Geometry check sheet. Reference: drawing and pictorial views, mm from the part's lowest x, y, z. A direction names the side the tool comes from. Coordinates: 2 decimals unless noted, no trailing zeros. Write each loop counter-clockwise with the first axis right and the second up, starting at its lowest first coordinate (ties: lowest second). Pieces come first, ordered by that corner, then holes. Notation, with made-up numbers: M -38,89 L 5,89 A31 cw 5,122 Z; hole C 49,-28.5 d11. An arc over 180 degrees is marked long. One line per item, written item: value.
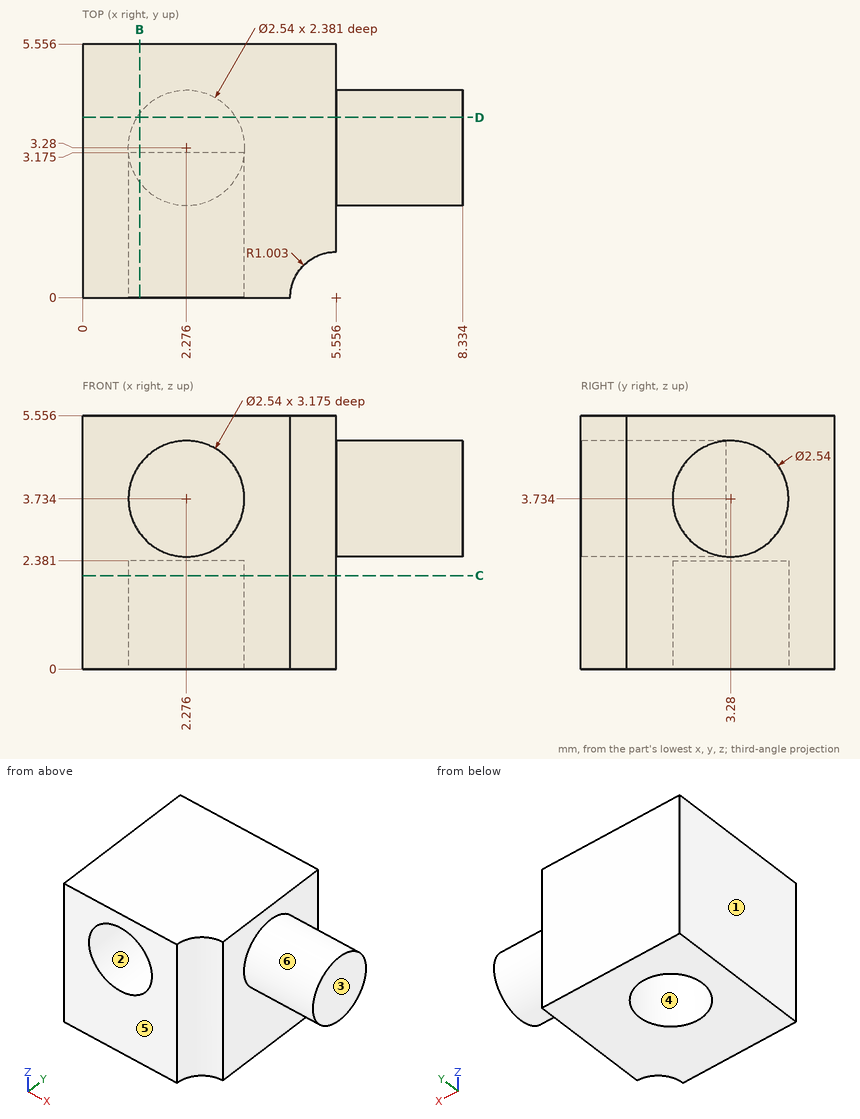
Item 1: Cross-section at D-D, the plane y = 3.95. Enter the section's corners in (x, z) (1 decimal).
The answers:
outline: M 0,0 L 1.2,0 L 1.2,2.4 L 3.4,2.4 L 3.4,0 L 5.6,0 L 5.6,2.7 L 8.3,2.7 L 8.3,4.8 L 5.6,4.8 L 5.6,5.6 L 0,5.6 Z
Item 2: Go/stop test with flat-tipped pins: P1, Ø1, axis at y = 5, z = 3.5, coming from the +X side; P2, Ø3, axis at y = 2.5, z = 1, coming from the +X side. Record where each tip stops, or that it passes through.
The answers:
P1: stops at x = 8.33
P2: stops at x = 5.56
Item 3: Scan lines: line 1 (Y direction, x = 3, z = 4.7) (1 decimal); line 2 (Y direction, x = 3.25, z = 2.2) (1 decimal); line 3 (X direction, y = 1.9, z = 4.35) (1 decimal). Record each from-to range of solid material in increasing order.
The answers:
line 1: y = 3.2 to 5.6
line 2: y = 0 to 2.5, 4.1 to 5.6
line 3: x = 0 to 1.2, 3.4 to 5.6
Item 4: Cross-section at B-B, the plane x = 1.25. Enter the section's corners in (y, z) (1 decimal).
The answers:
outline: M 0,0 L 2.5,0 L 2.5,2.4 L 4,2.4 L 4,0 L 5.6,0 L 5.6,5.6 L 0,5.6 L 0,4.5 L 3.2,4.5 L 3.2,3 L 0,3 Z
Item 5: Cross-section at C-C, the plane z = 2.05. Enter the section's corners in (x, y), and give its area (3 significant figures).
The answers:
outline: M 0,0 L 4.55,0 A1 cw 5.56,1 L 5.56,5.56 L 0,5.56 Z; hole C 2.28,3.28 d2.54
area: 25.0 mm²
Item 6: Draft check along X on the marked faces 1, 2 and 3. Enter one of: released by +X, released by -X, zero draft, split by the parting line, or undercut.
The answers:
face 1: released by -X
face 2: undercut
face 3: released by +X
Item 7: Access from +Z, -Z, +X, -X, +Y, -Y to the whole of each face (thin tool, end or side, straight path). Record for the marked faces 4, 5 and 6.
The answers:
face 4: -Z
face 5: +Z, -Z, +X, -X, -Y
face 6: +X
